Part print with two shaded views. Sizes in mm from the minimum x, y, z corner. Round coordinates to 2 decimals unless told otherwise and drop trailing zeros. Order: outer loops, then holes, each group sorted by start corner. A loop starts at its lowest first (then second) coordinate and runs counter-clockwise, first axis right, second up. Notation, with made-up numbers: (-20.5, 13) - (18.5, 13) arc R26 cw to (18.5, 46) - close; hole circle Ø2 at (-17, 72.25). An arc over 180 degrees is marked (long way). Write item = value, one per line.
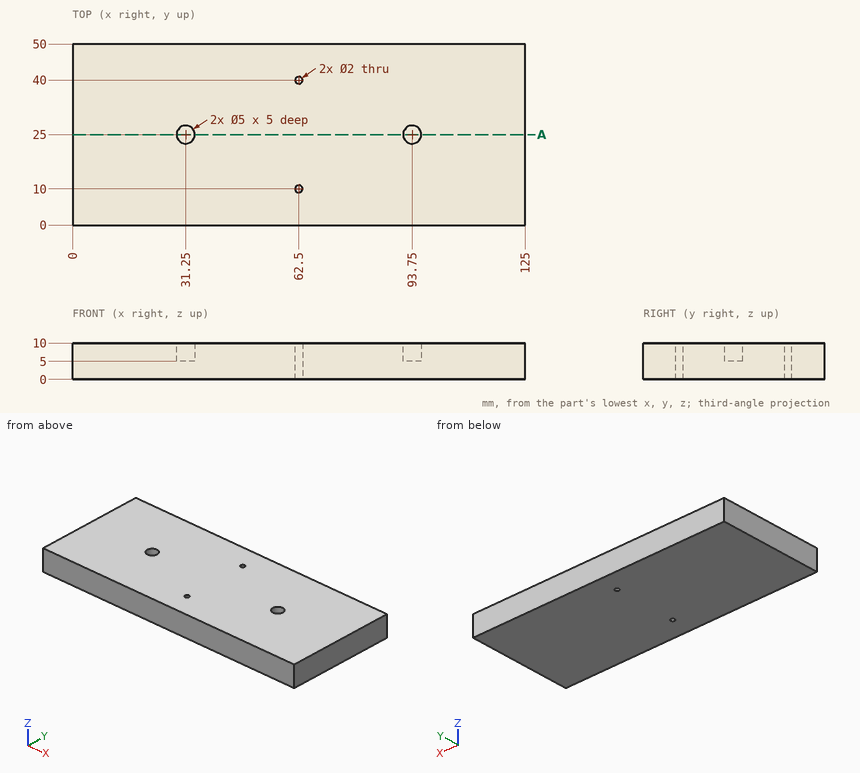
1) Cut at A-A (y = 25). Write the cut outline in (x, z).
Conclusion:
outline = (0, 0) - (125, 0) - (125, 10) - (96.25, 10) - (96.25, 5) - (91.25, 5) - (91.25, 10) - (33.75, 10) - (33.75, 5) - (28.75, 5) - (28.75, 10) - (0, 10) - close
2) Flat gauge pin, fed straight in: pin 1 Ø3 at (x, y) = (31.25, 25) entering from +Z. Where does the tip first touch, or does it go through?
Conclusion:
pin_1 = 5
3) Wall check: line 1 along Y through (x, z) = (62.5, 5.5); line 2 along X through (y, z) = (27, 6); line 3 along Y through (x, z) = (31.25, 8.55). Give the ranges that are in metal, low to high.
Conclusion:
line_1 = 0 to 9, 11 to 39, 41 to 50
line_2 = 0 to 29.75, 32.75 to 92.25, 95.25 to 125
line_3 = 0 to 22.5, 27.5 to 50
